from build123d import *

# Parameters (mm, degrees)
SKETCH_1_W      = 3
SKETCH_1_H      = 28
EXTRUDE_1_DEPTH = 5
SKETCH_2_W      = 11
SKETCH_2_H      = 36
EXTRUDE_2_DEPTH = 1.5
FILLET_1_R      = 1
FILLET_3_R      = 2
EXTRUDE_3_DEPTH = 2.9


with BuildPart() as part:
    # Эскиз1 → Бобышка-Вытянуть1 (new body)
    with BuildSketch(Plane(origin=(0, 0, 0), x_dir=(1, 0, 0), z_dir=(0, 1, 0))):
        Rectangle(SKETCH_1_W, SKETCH_1_H)
    extrude(amount=EXTRUDE_1_DEPTH)

    # Эскиз2 → Бобышка-Вытянуть2 (add)
    with BuildSketch(Plane.XZ):
        Rectangle(SKETCH_2_W, SKETCH_2_H)
    extrude(amount=EXTRUDE_2_DEPTH)

    # Скругление1
    fillet_1_edges = [part.edges().sort_by_distance(p)[0] for p in [
        (-1.5, 2.5, -14),
        (1.5, 2.5, -14),
        (1.5, 2.5, 14),
        (-1.5, 2.5, 14),
    ]]
    fillet(fillet_1_edges, radius=FILLET_1_R)

    # Скругление3
    fillet_3_edges = [part.edges().sort_by_distance(p)[0] for p in [
        (5.5, -0.75, -18),
        (5.5, -0.75, 18),
        (-5.5, -0.75, 18),
        (-5.5, -0.75, -18),
    ]]
    fillet(fillet_3_edges, radius=FILLET_3_R)

    # Эскиз3 → Бобышка-Вытянуть3 (add)
    with BuildSketch(Plane(origin=(0, 5, 0), x_dir=(1, 0, 0), z_dir=(0, 1, 0))):
        Polygon((-1.5, 0), (0, 1.5), (1.5, 0), (0, -1.5), align=None)
    extrude(amount=EXTRUDE_3_DEPTH)


solid = part.part
Build history of the part. All positions in model axes, mm. A direction names the side the tool comes from. Round coordinates to 2 decimals unless told otherwise and drop trailing zeros. Write each loop counter-clockwise with the first axis right and the second up, starting at its lowest first coordinate (ties: lowest second). Pieces come first, ordered by that corner, then holes. Notation, with made-up numbers: (-20.5, -14.75) -> (4.5, -14.75) arc R22 cw to (4.5, -8.75) -> close; hole circle Ø3 at (-10, 40). An arc over 180 degrees is marked (long way). Use one line per item in the form item = value.
Q1. Band-saw the part on D-D, the plane y = 6.5. Write the cut outline in (x, z), then the cut area to 3 significant figures.
Conclusion:
outline = (-1.5, 0) -> (0, -1.5) -> (1.5, 0) -> (0, 1.5) -> close
area = 4.50 mm²
Q2. Tool access for faces 1 (the cylindrical face through (-1.215, 2.535, 13.699)), 2 (the flat face through (-1.5, 2, 0)), 3 (the flat face through (1.5, 2, 0)): list every direction of +Z, -Z, +X, -X, +Y, -Y with a clear straight run to the whole face (end or side of a thin tool).
Conclusion:
face_1 = +Z, -X, +Y
face_2 = +Z, -Z, -X, +Y
face_3 = +Z, -Z, +X, +Y
Q3. Drill centre lines: L1, parallel to Y at x = 2, z = 13.5; L2, parallel to X at y = 1.25, z = -13; L3, parallel to Y at x = -1, z = 7. Where is each one in solid material? Low to high.
Conclusion:
L1 = -1.5 to 0
L2 = -1.5 to 1.5
L3 = -1.5 to 5
Q4. Band-saw the part on B-B, the plane y = 1.5. Write the cut outline in (x, z).
Conclusion:
outline = (-1.5, -13) arc R1 ccw to (-0.5, -14) -> (0.5, -14) arc R1 ccw to (1.5, -13) -> (1.5, 13) arc R1 ccw to (0.5, 14) -> (-0.5, 14) arc R1 ccw to (-1.5, 13) -> close
Q5. Drop flat-ended pins along their axis: P1, Ø1.5, axis at y = 3, z = 4, coming from the +X side; P2, Ø1, axis at y = 6, z = -9.5, coming from the -X side; P3, Ø4, axis at y = 2.5, z = 5.5, coming from the -X side; P4, Ø5.5, axis at x = -1, z = 1, coming from the +Y side. Give the stop position or say it passes through.
Conclusion:
P1 = 1.5
P2 = through
P3 = -1.5
P4 = 7.9
Q6. Band-saw the part on C-C, the plane x = -2. Write the cut outline in (y, z).
Conclusion:
outline = (-1.5, -18) -> (0, -18) -> (0, 18) -> (-1.5, 18) -> close
Q7. Band-saw the part on A-A, the plane z = -1. Write the cut outline in (x, y).
Conclusion:
outline = (-5.5, -1.5) -> (5.5, -1.5) -> (5.5, 0) -> (1.5, 0) -> (1.5, 5) -> (0.5, 5) -> (0.5, 7.9) -> (-0.5, 7.9) -> (-0.5, 5) -> (-1.5, 5) -> (-1.5, 0) -> (-5.5, 0) -> close
